Part model, mm, in its own coordinate system. Face numbers are marked on the shaded views. A direction names the side the tool comes from. Give positions to 0.01 mm unless a question says otherwise; leave off trailing zeros. Order: outer loops, then holes, each group sorted by start corner. A loop starts at its lowest first (then second) coordinate and runs counter-clockwise, first axis right, second up. Notation, with made-up numbers: (14.25, -29) - (51.25, -29) arc R8 cw to (51.25, -24) - close; hole circle Ø3 at (18, 78). An arc over 180 degrees is marked (long way). Use one line per item in the form item = value. Start each with the question number.
1. Band-saw the part on A-A, the plane x = 32. List the corners of the cut face in (y, z).
2. Pin check, flat tips, straight feed: P1, Ø1, axis at x = 13.5, y = 2.5, coming from the +Z side; P2, Ø2.5, axis at x = 45, y = 0, coming from the -Z side; P3, Ø3.5, axis at x = 52, y = 0, coming from the +Z side; P4, Ø3, axis at x = 2.5, z = 3.5, coming from the -Y side. Stop position of each tip, or through.
3. Drill centre lines: line 1 (Y direction, x = 0, z = 2.9); line 2 (X direction, y = -1, z = 1.2); line 3 (Z direction, x = 30, y = -0.5). Where is each one in solid material? Low to high.
4. Band-saw the part on D-D, the plane z = 3.85. List the corners of the cut face in (x, y), plus the area to 3 significant figures.
5. Band-saw the part on B-B, the plane z = 1. List the corners of the cut face in (x, y).
6. Tool access for the marked faces 1 and 2: list every direction of +Z, -Z, +X, -X, +Y, -Y with a clear straight run to the whole face (end or side of a thin tool).
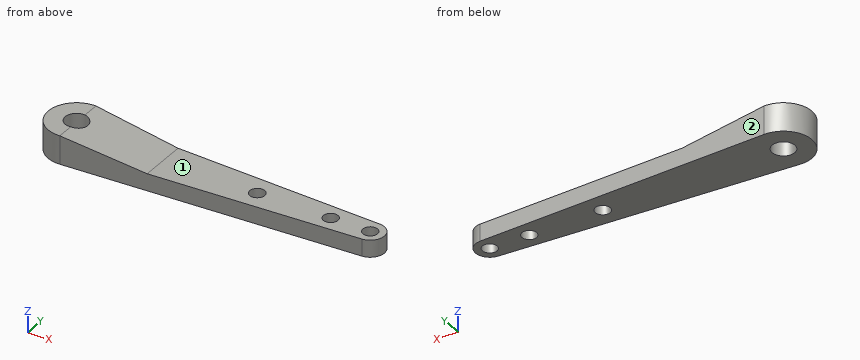
Autodesk Inventor part; units mm, degrees
ref_plane "YZ Plane" through (0, 0, 0) normal (1, 0, 0) x (0, 1, 0)
ref_plane "XZ Plane" through (0, 0, 0) normal (0, 1, 0) x (-1, 0, 0)
ref_plane "XY Plane" through (0, 0, 0) normal (0, 0, 1) x (1, 0, 0)
sketch "Skizze1" plane through (0, 0, 0) normal (0, 0, 1) x (1, 0, 0)
  line L0 (0, 7) -> (0, -7) construction
  line L1 (-16.9, 0) -> (66.4, 0) construction
  circle A0 centre (0, 0) radius 2
  circle A1 centre (32, 0) radius 1.3257
  circle A2 centre (45, 0) radius 1.3
  circle A3 centre (52, 0) radius 1.3
  arc A4 (52.1202, -2.4971) -> (52.1202, 2.4971) centre (52, 0) ccw
  arc A5 (0.2404, 4.9942) -> (0.2404, -4.9942) centre (0, 0) ccw
  line L2 (0.2404, 4.9942) -> (52.1202, 2.4971)
  line L3 (0.2404, -4.9942) -> (52.1202, -2.4971)
  line L4 (0.2404, -4.9942) -> (0.2404, -1.9855)
  line L5 (0.2404, 1.9855) -> (0.2404, 4.9942)
  line L6 (0.2404, 1.9855) -> (0.2404, -1.9855)
  dimension "d0" = 32
  dimension "d1" = 45
  dimension "d2" = 52
  dimension "d3" = 5
  dimension "d4" = 2.6
  dimension "d5" = 4
  dimension "d6" = 10
extrude "Extrusion1" add sketch "Skizze1" along normal blind 3
extrude "Extrusion2" add sketch "Skizze1" along normal blind 5 contours L6 A0 | A0 L4 A5 L5 picked at (-1.282, 0.0747)
chamfer "Fase1" distance 15 distance2 2 1 edges at (0.2404, 0, 3) measured on face at (10.385, 0, 3)
extrude "Extrusion3" cut sketch "Skizze1" along normal blind 5 contours A0 L6 | L6 A0
properties part number "Servo-Arm-52mm"
From the geometry:
q1.outline = (-3.47, 0) - (-1.33, 0) - (-1.33, 3) - (-3.47, 3) - close; (1.33, 0) - (3.47, 0) - (3.47, 3) - (1.33, 3) - close
q2.P1 = 3.3
q2.P2 = through
q2.P3 = 3
q2.P4 = -4.96
q3.line_1 = -5 to -2, 2 to 5
q3.line_2 = -4.9 to -1.73, 1.73 to 31.13, 32.87 to 44.17, 45.83 to 51.17, 52.83 to 54.29
q3.line_3 = 0 to 3
q4.outline = (0.24, -4.99) - (8.86, -4.58) - (8.86, 4.58) - (0.24, 4.99) arc R5 ccw (long way) to start; hole circle Ø4 at (0, 0)
q4.area = 112 mm²
q5.outline = (0.24, -4.99) - (52.12, -2.5) arc R2.5 ccw to (52.12, 2.5) - (0.24, 4.99) arc R5 ccw (long way) to start; hole circle Ø4 at (0, 0); hole circle Ø2.65 at (32, 0); hole circle Ø2.6 at (45, 0); hole circle Ø2.6 at (52, 0)
q6.face_1 = +Z, +X, +Y, -Y
q6.face_2 = +Z, -Z, +X, +Y
